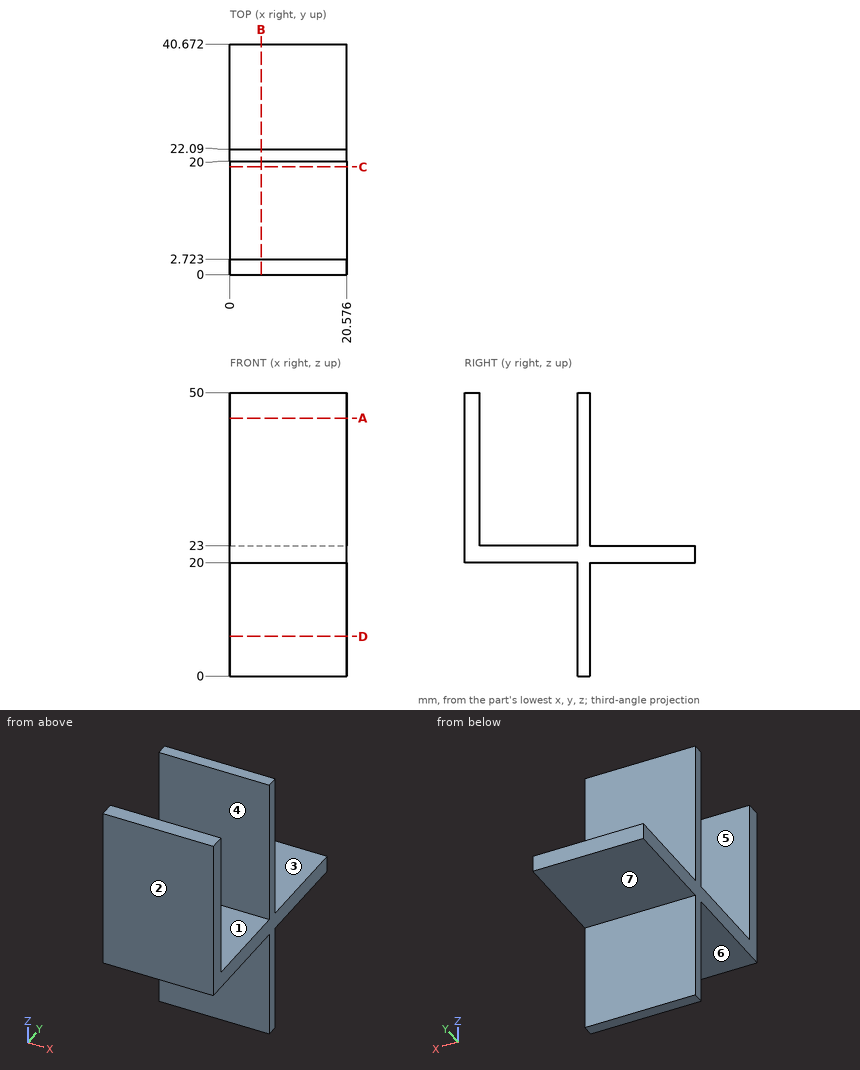
Check sheet for the drawn part. Datum: minimum x, y, z corner. Units: mm. A direction names the side the tool comes from. Coordinates: 2 decimals unless noted, no trailing zeros. Write each loop counter-clockwise with the first axis right and the second up, starting at its lowest first coordinate (ties: lowest second). Pieces come first, ordered by that corner, then holes. Notation, with made-up numbers: (75, 26.25) - (91, 26.25) arc R26 ccw to (91, 52.25) - close; hole circle Ø8 at (-32, -14.75). An arc over 180 degrees is marked (long way). Answer as a JSON object with one key per item and string values.
(1) Cross-section at B-B on x = 5.5. Record the cut outline in (y, z), plus the area to 3 significant figures.
Report:
{"outline": "(0, 20) - (20, 20) - (20, 0) - (22.09, 0) - (22.09, 20) - (40.67, 20) - (40.67, 23) - (22.09, 23) - (22.09, 50) - (20, 50) - (20, 23) - (2.72, 23) - (2.72, 50) - (0, 50) - close", "area": "294 mm^2"}
(2) Cross-section at A-A on z = 45.5. Record the cut outline in (x, y).
Report:
{"outline": "(0, 0) - (20.58, 0) - (20.58, 2.72) - (0, 2.72) - close; (0, 20) - (20.58, 20) - (20.58, 22.09) - (0, 22.09) - close"}
(3) Tool access check on the marked faces 5, 6 and 7. Record the directions out of +Z, -Z, +X, -X, +Y, -Y that give a thin tool (end or side, any length) a straight path to the whole face; none if there is none.
Report:
{"face 5": "+Z, +X, -X", "face 6": "-Z, +X, -X, -Y", "face 7": "-Z, +X, -X, +Y"}
(4) Mould release check, pull along Y, two halves, no side actions. Record for the marked faces 1, 2, 3 and 4: pulls with the +Y half, pulls with the -Y half, needs draft (parallel to the pull), parting line crosses it, or undercut.
Report:
{"face 1": "undercut", "face 2": "pulls with the -Y half", "face 3": "needs draft", "face 4": "undercut"}
(5) Gauge pin test, flat ends, axial feed: pin 1 Ø1.5 at (x, y) = (12, 4.5) entering from -Z; pin 2 Ø6 at (x, z) = (8.5, 31.5) entering from +Y; pin 3 Ø8.5 at (x, y) = (11, 9) entering from +Z; pin 4 Ø10 at (y, z) = (33, 26.5) entering from -X. Record the tip position at first contact, or that the pin passes through.
Report:
{"pin 1": "z = 20", "pin 2": "y = 22.09", "pin 3": "z = 23", "pin 4": "x = 0"}
(6) Cross-section at D-D on z = 7. Record the cut outline in (x, y).
Report:
{"outline": "(0, 20) - (20.58, 20) - (20.58, 22.09) - (0, 22.09) - close"}
(7) Cross-section at C-C on y = 19. Record the cut outline in (x, z).
Report:
{"outline": "(0, 20) - (20.58, 20) - (20.58, 23) - (0, 23) - close"}
(8) Thickness scan on line 1 along Y through (x, z) = (9.25, 28.5); line 2 along Z through (x, y) = (17, 24); line 3 along Y through (x, z) = (11.5, 9.5). Record the ranges inside material, lowest first.
Report:
{"line 1": "0 to 2.72, 20 to 22.09", "line 2": "20 to 23", "line 3": "20 to 22.09"}
